Part model, mm, in its own coordinate system. A direction names the side the tool comes from. Coordinates: 2 decimals unless noted, no trailing zeros. Order: outer loops, then holes, each group sorted by start corner. A loop starts at its lowest first (then second) coordinate and runs counter-clockwise, first axis right, second up.
```python
from build123d import *

# Parameters (mm, degrees)
F0_W     = 76.2
F0_H     = 139.7
F1_DEPTH = 7.62
F2_W     = 76.2
F2_H     = 12.7
F3_DEPTH = 12.7
F4_R     = 7.988777
F5_DEPTH = 12.7


with BuildPart() as f1:
    # F0 (on Front) → F1 (new body)
    with BuildSketch(Plane.XZ):
        Rectangle(F0_W, F0_H)
    extrude(amount=F1_DEPTH)

    # F2 (on face) → F3 (join)
    with BuildSketch(Plane.XZ.offset(7.62)):
        with Locations((0, -63.5)):
            Rectangle(F2_W, F2_H)
    extrude(amount=F3_DEPTH)

    # F4 (on face) → F5 (cut)
    with BuildSketch(Plane(origin=(0, 0, -69.85), x_dir=(1, 0, 0), z_dir=(0, 0, -1))):
        with Locations((0, 10.788938)):
            Circle(F4_R)
    extrude(amount=-F5_DEPTH, mode=Mode.SUBTRACT)


solid = f1.part
```
(1) Slice it at C-C, the plane z = 32.5. Give the cut face in (x, y), then the cut area to 3 significant figures.
(2) Pull direction X, two halves, no side cores. Call faces 4 (the face through (-38.1, -6, -17)), 5 (the face through (-7.98, -11.14, -63.59)), 6 (the face through (-9, -10, -69.85)), 7 (the face through (38.1, -6, -17)): +X half, -X half, draft (parallel to the pull), parting line (faces both ways), or undercut.
(3) Probe line 1 (Y direction, x = 0, z = -61.75); line 2 (Y direction, x = -23.5, z = -30); line 3 (X direction, y = -4, z = -60). List the from-to ranges inside material, lowest first.
(4) Slice it at A-A, the plane x = 0. Give the cut face in (y, z).
(5) Tool access for faces 1 (the face through (-1, -7.62, 7)), 2 (the face through (-1, -20.32, -63)), 3 (the face through (0, -6, -57.15)): list every direction of +Z, -Z, +X, -X, +Y, -Y with a clear straight run to the whole face (end or side of a thin tool).
(6) Slice it at D-D, the plane x = 31. Give the cut face in (y, z), then the cut area to 3 significant figures.
(7) Drop flat-ended pins along their axis: pin 1 (10 mm diameter, centred on x = 10.5, y = -11, fed in from +Z); pin 2 (6 mm diameter, centred on x = -20.5, y = -17.5, fed in from +Z); pin 3 (2.5 mm diameter, centred on x = 1.5, y = -5.5, fed in from -Z). Give the stop position or say it passes through.
(8) Slice it at B-B, the plane y = -6.25. Give the cut face in (x, z).
Here are the results:
1. outline: (-38.1, -7.62) - (38.1, -7.62) - (38.1, 0) - (-38.1, 0) - close
1. area: 581 mm2
2. face 4: -X half
2. face 5: undercut
2. face 6: draft
2. face 7: +X half
3. line 1: y = -20.32 to -18.78, -2.8 to 0
3. line 2: y = -7.62 to 0
3. line 3: x = -38.1 to -4.21, 4.21 to 38.1
4. outline: (-20.32, -69.85) - (-18.78, -69.85) - (-18.78, -57.15) - (-20.32, -57.15) - close; (-7.62, -57.15) - (-2.8, -57.15) - (-2.8, -69.85) - (0, -69.85) - (0, 69.85) - (-7.62, 69.85) - close
5. face 1: +Z, +X, -X, -Y
5. face 2: +Z, -Z, +X, -X, -Y
5. face 3: -Z
6. outline: (-20.32, -69.85) - (0, -69.85) - (0, 69.85) - (-7.62, 69.85) - (-7.62, -57.15) - (-20.32, -57.15) - close
6. area: 1,230 mm2
7. pin 1: stops at z = 69.85
7. pin 2: stops at z = -57.15
7. pin 3: stops at z = -57.15
8. outline: (-38.1, -69.85) - (-6.57, -69.85) - (-6.57, -57.15) - (6.57, -57.15) - (6.57, -69.85) - (38.1, -69.85) - (38.1, 69.85) - (-38.1, 69.85) - close
